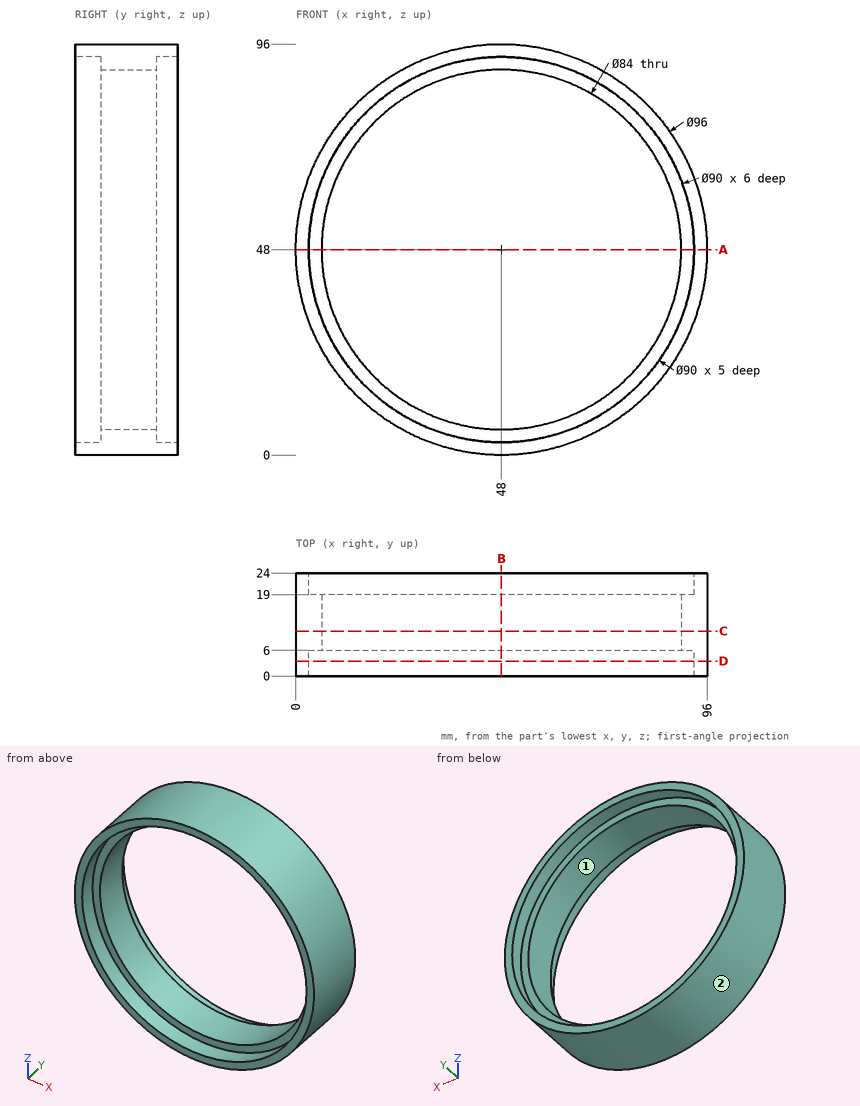
Drawing for the job (mm, zero at the part's lowest x, y, z). Give positions to 0.01 mm unless a question says otherwise; leave off trailing zeros. Write each loop counter-clockwise with the first axis right and the second up, starting at its lowest first coordinate (ties: lowest second). Pieces come first, ordered by that corner, then holes. Notation, with made-up numbers: M 86.25,11 L 142.25,11 A20 cw 142.25,33 Z; hole C -9.75,44 d9. An arc over 180 degrees is marked long. Return JSON: item names as keys, results as strings. Group by question number.
(1) Band-saw the part on C-C (y = 10.5). Give the cut face in (x, z).
(2) Band-saw the part on A-A (z = 48). Give the cut face in (x, y).
(3) Mould opens along X. For the marked faces 1 and 2 say: pulls with the +X half, pulls with the -X half, needs draft (parallel to the pull), parting line crosses it, or undercut.
(4) Band-saw the part on B-B (x = 48). Give the cut face in (y, z), and give its area (3 significant figures).
(5) Drill centre lines: L1, parallel to X at y = 21.1, z = 48; L2, parallel to Z at x = 85.5, y = 18.25; L3, parallel to X at y = 3.25, z = 16. Where is each one in solid material? Low to high. Write a range as [from, to].
(6) Flat gauge pins, fed straight in: pin 1 Ø8 at (y, z) = (20, 81) entering from -X; pin 2 Ø2 at (x, y) = (13.5, 4) entering from -Z; pin 3 Ø6 at (x, y) = (54, 12) entering from -Z; pin 4 Ø10 at (x, z) = (16.5, 57.5) entering from -Y. Where does each tip first touch, or does it go through?
(7) Band-saw the part on D-D (y = 3.5). Give the cut face in (x, z).
Entries:
{
 "1": {"outline": "C 48,48 d96; hole C 48,48 d84"},
 "2": {"outline": "M 0,0 L 3,0 L 3,6 L 6,6 L 6,19 L 3,19 L 3,24 L 0,24 Z; M 90,6 L 93,6 L 93,0 L 96,0 L 96,24 L 93,24 L 93,19 L 90,19 Z"},
 "3": {"face 1": "undercut", "face 2": "parting line crosses it"},
 "4": {"outline": "M 0,0 L 24,0 L 24,3 L 19,3 L 19,6 L 6,6 L 6,3 L 0,3 Z; M 0,93 L 6,93 L 6,90 L 19,90 L 19,93 L 24,93 L 24,96 L 0,96 Z", "area": "222 mm^2"},
 "5": {"L1": "x = [0, 3], [93, 96]", "L2": "z = [18.04, 29.09], [66.91, 77.96]", "L3": "x = [12.22, 16.36], [79.64, 83.78]"},
 "6": {"pin 1": "stops at x = 9.75", "pin 2": "stops at z = 13.62", "pin 3": "stops at z = 0.09", "pin 4": "passes through"},
 "7": {"outline": "C 48,48 d96; hole C 48,48 d90"}
}
